from build123d import *

# Parameters (mm, degrees)
SKETCH1_W               = 49
SKETCH1_H               = 60
BOSS_EXTRUDE1_DEPTH     = 15
SKETCH5_W               = 6.5
SKETCH5_H               = 13
CUT_EXTRUDE2_DEPTH      = 54
SKETCH2_R               = 1.5
CUT_EXTRUDE3_DEPTH      = 54
SKETCH7_W               = 6.5
SKETCH7_H               = 13
CUT_EXTRUDE4_DEPTH      = 54
SKETCH8_W               = 29
SKETCH8_H               = 1.5
CUT_EXTRUDE5_DEPTH      = 54
SKETCH9_W               = 29
SKETCH9_H               = 1.5
CUT_EXTRUDE6_DEPTH      = 54
CUT_EXTRUDE7_DEPTH      = 17
CUT_EXTRUDE7_DEPTH_BACK = 76
SKETCH14_W              = 29
SKETCH14_H              = 1.5
SKETCH16_W              = 29
SKETCH16_H              = 1.5
CUT_EXTRUDE8_DEPTH      = 17
SKETCH17_W              = 29
SKETCH17_H              = 0.5
CUT_EXTRUDE9_DEPTH      = 7
SKETCH18_W              = 29
SKETCH18_H              = 0.5
CUT_EXTRUDE10_DEPTH     = 7
SKETCH19_W              = 42.757359313
SKETCH19_H              = 4.257359312
CUT_EXTRUDE12_DEPTH     = 51


with BuildPart() as part:
    # Sketch1 → Boss-Extrude1 (new body)
    with BuildSketch(Plane(origin=(0, 0, 0), x_dir=(1, 0, 0), z_dir=(0, 1, 0))):
        with Locations((-27.855953383, 4.497926564)):
            Rectangle(SKETCH1_W, SKETCH1_H)
    extrude(amount=BOSS_EXTRUDE1_DEPTH)

    # Sketch5 → Cut-Extrude2 (cut)
    with BuildSketch(Plane.ZY.offset(52.355953383)):
        with Locations((-31.247926564, 8.5)):
            Rectangle(SKETCH5_W, SKETCH5_H)
    extrude(amount=-CUT_EXTRUDE2_DEPTH, mode=Mode.SUBTRACT)

    # Sketch2 → Cut-Extrude3 (cut)
    with BuildSketch(Plane(origin=(0, 15, 0), x_dir=(-1, 0, 0), z_dir=(0, 1, 0))):
        with Locations(Location((45.355953383, -31.247926564, 0), (0, 0, 270))):
            Circle(SKETCH2_R)
        with Locations(Location((10.355953383, -31.247926564, 0), (0, 0, 270))):
            Circle(SKETCH2_R)
        with Locations(Location((10.355953383, 22.252073436, 0), (0, 0, 90))):
            Circle(SKETCH2_R)
        with Locations(Location((45.355953383, 22.252073436, 0), (0, 0, 90))):
            Circle(SKETCH2_R)
    extrude(amount=-CUT_EXTRUDE3_DEPTH, mode=Mode.SUBTRACT)

    # Sketch7 → Cut-Extrude4 (cut)
    with BuildSketch(Plane.ZY.offset(52.355953383)):
        with Locations((22.252073436, 8.5)):
            Rectangle(SKETCH7_W, SKETCH7_H)
    extrude(amount=-CUT_EXTRUDE4_DEPTH, mode=Mode.SUBTRACT)

    # Sketch8 → Cut-Extrude5 (cut)
    with BuildSketch(Plane.XY.offset(19.002073436)):
        Polygon((-52.355953383, 8.5), (-42.355953383, 8.5), (-13.355953383, 8.5), (-3.355953383, 8.5), (-3.355953383, 15), (-52.355953383, 15), align=None)
        with Locations((-27.855953383, 7.75)):
            Rectangle(SKETCH8_W, SKETCH8_H)
    extrude(amount=-CUT_EXTRUDE5_DEPTH, mode=Mode.SUBTRACT)

    # Sketch9 → Cut-Extrude6 (cut)
    with BuildSketch(Plane(origin=(0, 7, 0), x_dir=(-1, 0, 0), z_dir=(0, 1, 0))):
        with Locations((27.855953383, -27.247926564)):
            Rectangle(SKETCH9_W, SKETCH9_H)
    extrude(amount=-CUT_EXTRUDE6_DEPTH, mode=Mode.SUBTRACT)

    # Sketch14 → Cut-Extrude7 (cut, two sides: drawn at the far end of the back side and taken through both)
    with BuildSketch(Plane(origin=(0, 0, -26.497926564), x_dir=(-1, 0, 0), z_dir=(0, 0, -1)).offset(-CUT_EXTRUDE7_DEPTH_BACK)):
        with Locations((27.855953383, 0.75)):
            Rectangle(SKETCH14_W, SKETCH14_H)
    extrude(amount=CUT_EXTRUDE7_DEPTH + CUT_EXTRUDE7_DEPTH_BACK, mode=Mode.SUBTRACT)

    # Sketch16 → Cut-Extrude8 (cut)
    with BuildSketch(Plane(origin=(0, 7, 0), x_dir=(-1, 0, 0), z_dir=(0, 1, 0))):
        with Locations((27.855953383, 18.252073436)):
            Rectangle(SKETCH16_W, SKETCH16_H)
    extrude(amount=-CUT_EXTRUDE8_DEPTH, mode=Mode.SUBTRACT)

    # Sketch17 → Cut-Extrude9 (cut)
    with BuildSketch(Plane.XY.offset(25.502073436)):
        with Locations((-27.855953383, 1.75)):
            Rectangle(SKETCH17_W, SKETCH17_H)
    extrude(amount=-CUT_EXTRUDE9_DEPTH, mode=Mode.SUBTRACT)

    # Sketch18 → Cut-Extrude10 (cut)
    with BuildSketch(Plane(origin=(0, 0, -34.497926564), x_dir=(-1, 0, 0), z_dir=(0, 0, -1))):
        with Locations((27.855953383, 1.75)):
            Rectangle(SKETCH18_W, SKETCH18_H)
    extrude(amount=-CUT_EXTRUDE10_DEPTH, mode=Mode.SUBTRACT)

    # Sketch19 → Cut-Extrude12 (cut)
    with BuildSketch(Plane.ZY.offset(52.355953383)):
        with Locations((-4.497926565, 4.25)):
            Rectangle(SKETCH19_W, SKETCH19_H)
    extrude(amount=-CUT_EXTRUDE12_DEPTH, mode=Mode.SUBTRACT)


solid = part.part
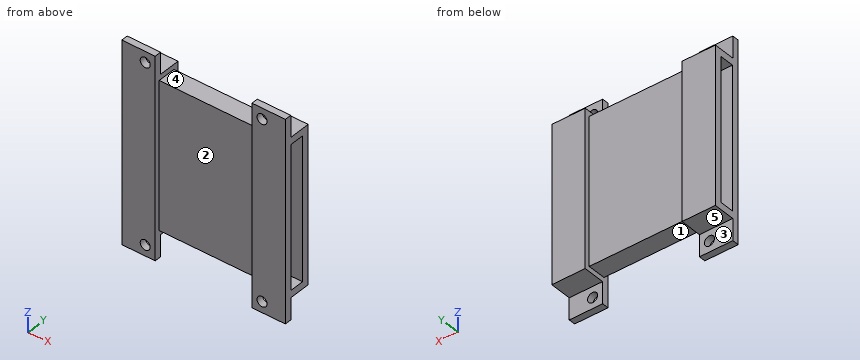
Source: CAD feature listing. Evaluate the final solid. Frame: model axes, mm. Face numbers are marked on the shaded views. A direction names the side the tool comes from. Coordinates: 2 decimals unless noted, no trailing zeros. Loops run counter-clockwise (first coordinate to the right, second up) from the corner with the lowest first, then second, coordinate; pieces in that order, holes last. Notation, with made-up numbers: (84, -16) - (124, -16) arc R30 cw to (124, 14) - close; hole circle Ø10 at (37, 52.25). An arc over 180 degrees is marked (long way). Return JSON: item names as keys, results as strings.
Q1. Section A-A, the plane z = -5. Return loops of the section in (x, y).
Results:
{"outline": "(-52.36, 0) - (-42.36, 0) - (-42.36, 1.5) - (-13.36, 1.5) - (-13.36, 0) - (-3.36, 0) - (-3.36, 2.12) - (-52.36, 2.12) - close; (-52.36, 6.38) - (-3.36, 6.38) - (-3.36, 8.5) - (-13.36, 8.5) - (-13.36, 7) - (-42.36, 7) - (-42.36, 8.5) - (-52.36, 8.5) - close"}
Q2. Section C-C, the plane x = -25.5. Return loops of the section in (y, z), plus the area to 3 significant figures.
Results:
{"outline": "(1.5, -26.5) - (7, -26.5) - (7, 17.5) - (1.5, 17.5) - close; hole (2.12, -25.88) - (6.38, -25.88) - (6.38, 16.88) - (2.12, 16.88) - close", "area": "60.0 mm2"}
Q3. Mould query, pull axis X, two halves, no side actions, for the marked faces 4 and 5. Classes: released by +X, released by -X, zero draft, split by the parting line, or undercut.
Results:
{"face 4": "undercut", "face 5": "zero draft"}
Q4. Material intervals for line 1 along Y through (x, z) = (-47, -12.5); line 2 along Z through (x, y) = (-42, 6); line 3 along Z through (x, y) = (-49.5, 5), sorted ascending.
Results:
{"line 1": "0 to 2.12, 6.38 to 8.5", "line 2": "-26.5 to -25.88, 16.88 to 17.5", "line 3": "-28 to -25.88, 16.88 to 19"}
Q5. Access query for the marked faces 1, 2 and 3. Directions: +Z, -Z, +X, -X, +Y, -Y. A direction counts if a zero-diameter tool reaches every point of the face in a straight line with its end or side. Return the directions, or none.
Results:
{"face 1": "-Z, +Y, -Y", "face 2": "+Z, -Z, -Y", "face 3": "-Z, +X, -X, +Y"}
Q6. Contact query for flat-ended pins moving along their axis: P1, Ø3, axis at x = -45.5, z = -30.5, coming from the +Y side; P2, Ø8.5, axis at x = -31, z = -14.5, coming from the +Y side; P3, Ø3, axis at x = -6.5, y = 5, coming from the -Z side; P4, Ø2.5, axis at x = -45.36, z = 22.25, coming from the -Y side. Output: stop coordinate, or through.
Results:
{"P1": "y = 2", "P2": "y = 7", "P3": "z = -28", "P4": "through"}
Q7. Section B-B, the plane y = 3. Return loops of the section in (x, z).
Results:
{"outline": "(-52.36, -28) - (-42.36, -28) - (-42.36, -26.5) - (-13.36, -26.5) - (-13.36, -28) - (-3.36, -28) - (-3.36, -25.88) - (-52.36, -25.88) - close; (-52.36, 16.88) - (-3.36, 16.88) - (-3.36, 19) - (-13.36, 19) - (-13.36, 17.5) - (-42.36, 17.5) - (-42.36, 19) - (-52.36, 19) - close"}
